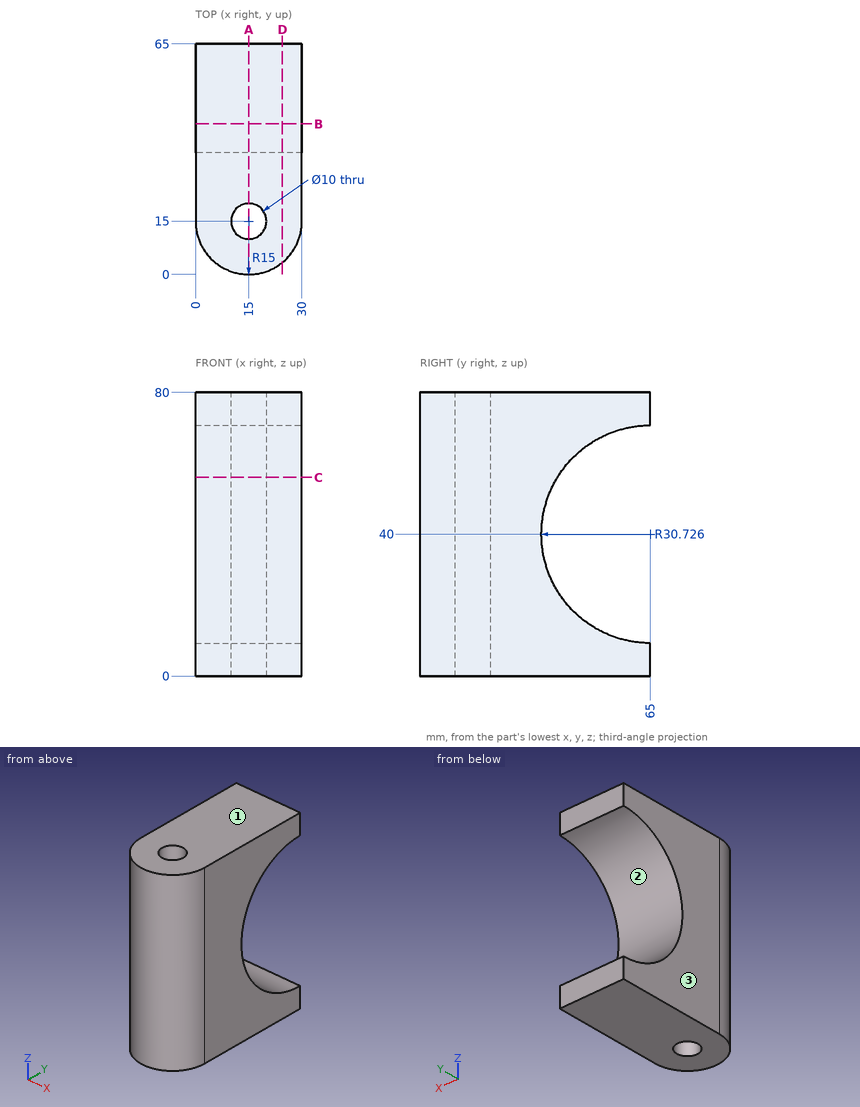
Answer from the drawing. Dimensions are ordinates in mm from the lowest x, y and z of the part. Give positions to 0.01 mm unless a question says otherwise; leave off trailing zeros. Order: outer loops, then holes, each group sorted by start corner. A loop starts at its lowest first (then second) coordinate and runs counter-clockwise, first axis right, second up. Notation, with made-up numbers: (76.5, -6.75) -> (131.5, -6.75) arc R37 cw to (131.5, 32.25) -> close; hole circle Ø7 at (70, 2.25). An arc over 180 degrees is marked (long way). Answer as a JSON object with one key per item and string values. Group by question number.
1. Consider line 1 along Z through (x, y) = (8.25, 56); line 2 along Y through (x, z) = (15, 43); line 3 along Z through (x, y) = (8, 47.5) (1 decimal). Determine where each line is inside the solid, lowest interval first. Write a range as [from, to].
2. The mould has two halves that part along Z. Classify the marked faces 1, 2 and 3: released by +Z, released by -Z, zero draft, split by the parting line, or undercut.
3. Section C-C on z = 56 is taken. Determine the outline of the cut face in (x, y).
4. Flat-ended cylindrical pins translate along their axes: pin 1 Ø3 at (x, z) = (7.5, 55) entering from +Y; pin 2 Ø2 at (y, z) = (12, 16) entering from +X; pin 3 Ø1 at (x, z) = (17.5, 24.5) entering from +Y; pin 4 Ø9 at (x, y) = (15, 15) entering from +Z. Find the tip coordinate at first contact, or state that the pin passes through.
5. Section D-D on x = 24.5 is taken. Determine the outline of the cut face in (y, z) (1 decimal), plus the area to 3 significant figures.
6. Section B-B on y = 42.5 is taken. Determine the outline of the cut face in (x, z).
7. Section A-A on x = 15 is taken. Determine the outline of the cut face in (y, z) (1 decimal).
Result sheet:
{
 "1": {"line 1": "z = [0, 10.62], [69.38, 80]", "line 2": "y = [0, 10], [20, 34.42]", "line 3": "z = [0, 14.7], [65.3, 80]"},
 "2": {"face 1": "released by +Z", "face 2": "undercut", "face 3": "zero draft"},
 "3": {"outline": "(0, 15) arc R15 ccw to (30, 15) -> (30, 38.77) -> (0, 38.77) -> close; hole circle Ø10 at (15, 15)"},
 "4": {"pin 1": "stops at y = 39.08", "pin 2": "stops at x = 29.87", "pin 3": "stops at y = 38.77", "pin 4": "passes through"},
 "5": {"outline": "(3.4, 0) -> (65, 0) -> (65, 9.3) arc R30.7 cw to (65, 70.7) -> (65, 80) -> (3.4, 80) -> close", "area": "3,450 mm^2"},
 "6": {"outline": "(0, 0) -> (30, 0) -> (30, 19.08) -> (0, 19.08) -> close; (0, 60.92) -> (30, 60.92) -> (30, 80) -> (0, 80) -> close"},
 "7": {"outline": "(0, 0) -> (10, 0) -> (10, 80) -> (0, 80) -> close; (20, 0) -> (65, 0) -> (65, 9.3) arc R30.7 cw to (65, 70.7) -> (65, 80) -> (20, 80) -> close"}
}
